```python
from build123d import *

# Parameters (mm, degrees)
BOSS_EXTRUDE1_DEPTH                             = 187.5
CUT_EXTRUDE1_DEPTH                              = 255
CUT_EXTRUDE2_DEPTH                              = 10
SKETCH4_R                                       = 1.5
CUT_EXTRUDE3_DEPTH                              = 255
SKETCH5_R                                       = 1.5
CUT_EXTRUDE4_DEPTH                              = 10
CSK_FOR_M3_FLAT_HEAD_MACHINE_SCREW1_D           = 3.4
CSK_FOR_M3_FLAT_HEAD_MACHINE_SCREW1_CSINK_D     = 6.3
CSK_FOR_M3_FLAT_HEAD_MACHINE_SCREW1_CSINK_ANGLE = 90
CSK_FOR_M3_FLAT_HEAD_MACHINE_SCREW2_D           = 3.4
CSK_FOR_M3_FLAT_HEAD_MACHINE_SCREW2_DEPTH       = 10
CSK_FOR_M3_FLAT_HEAD_MACHINE_SCREW2_CSINK_D     = 6.3
CSK_FOR_M3_FLAT_HEAD_MACHINE_SCREW2_CSINK_ANGLE = 90
CSK_FOR_M3_FLAT_HEAD_MACHINE_SCREW2_TIP         = 1.021463052
CSK_FOR_M3_FLAT_HEAD_MACHINE_SCREW3_D           = 3.4
CSK_FOR_M3_FLAT_HEAD_MACHINE_SCREW3_DEPTH       = 10
CSK_FOR_M3_FLAT_HEAD_MACHINE_SCREW3_CSINK_D     = 6.3
CSK_FOR_M3_FLAT_HEAD_MACHINE_SCREW3_CSINK_ANGLE = 90
CSK_FOR_M3_FLAT_HEAD_MACHINE_SCREW3_TIP         = 1.021463052


with BuildPart() as part:
    # Sketch1 → Boss-Extrude1 (new body, symmetric)
    with BuildSketch(Plane(origin=(0, 0, 0), x_dir=(0, 0, -1), z_dir=(1, 0, 0))):
        with BuildLine():
            Line((125, -45), (127, -45))
            Line((127, -45), (127, -2.5))
            ThreePointArc((127, -2.5), (126.267766953, -0.732233047), (124.5, 0))
            Line((124.5, 0), (-124.5, 0))
            ThreePointArc((-124.5, 0), (-126.267766953, -0.732233047), (-127, -2.5))
            Line((-127, -2.5), (-127, -45))
            Line((-127, -45), (-125, -45))
            Line((-125, -45), (-125, -2.5))
            ThreePointArc((-125, -2.5), (-124.853553391, -2.146446609), (-124.5, -2))
            Line((-124.5, -2), (124.5, -2))
            ThreePointArc((124.5, -2), (124.853553391, -2.146446609), (125, -2.5))
            Line((125, -2.5), (125, -45))
        make_face()
    extrude(amount=BOSS_EXTRUDE1_DEPTH, both=True)

    # Sketch2 → Cut-Extrude1 (cut, through all)
    with BuildSketch(Plane.XY.offset(127)):
        with BuildLine():
            Line((-169.5, -45), (169.5, -45))
            Line((169.5, -45), (169.5, -30))
            ThreePointArc((169.5, -30), (166.571067812, -22.928932188), (159.5, -20))
            Line((159.5, -20), (-159.5, -20))
            ThreePointArc((-159.5, -20), (-166.571067812, -22.928932188), (-169.5, -30))
            Line((-169.5, -30), (-169.5, -45))
        make_face()
    extrude(amount=-CUT_EXTRUDE1_DEPTH, mode=Mode.SUBTRACT)

    # Sketch3 → Cut-Extrude2 (cut)
    with BuildSketch(Plane(origin=(0, 0, 0), x_dir=(1, 0, 0), z_dir=(0, 1, 0))):
        with BuildLine():
            Line((-139.5, 97), (73.5, 97))
            ThreePointArc((73.5, 97), (80.571067812, 94.071067812), (83.5, 87))
            Line((83.5, 87), (83.5, -87))
            ThreePointArc((83.5, -87), (80.571067812, -94.071067812), (73.5, -97))
            Line((73.5, -97), (-139.5, -97))
            ThreePointArc((-139.5, -97), (-146.571067812, -94.071067812), (-149.5, -87))
            Line((-149.5, -87), (-149.5, 87))
            ThreePointArc((-149.5, 87), (-146.571067812, 94.071067812), (-139.5, 97))
        make_face()
    extrude(amount=-CUT_EXTRUDE2_DEPTH, mode=Mode.SUBTRACT)

    # Sketch4 → Cut-Extrude3 (cut, through all)
    with BuildSketch(Plane.XY.offset(127)):
        with Locations((-178.5, -33)):
            Circle(SKETCH4_R)
        with Locations((-166.5, -9)):
            Circle(SKETCH4_R)
        with Locations((166.5, -9)):
            Circle(SKETCH4_R)
        with Locations((178.5, -33)):
            Circle(SKETCH4_R)
    extrude(amount=-CUT_EXTRUDE3_DEPTH, mode=Mode.SUBTRACT)

    # Sketch5 → Cut-Extrude4 (cut)
    with BuildSketch(Plane(origin=(0, 0, 0), x_dir=(1, 0, 0), z_dir=(0, 1, 0))):
        with Locations(Location((-178.5, 118, 0), (0, 0, 270))):  # turned: the seam where the file's is
            Circle(SKETCH5_R)
        with Locations(Location((-154.5, 118, 0), (0, 0, 270))):  # turned: the seam where the file's is
            Circle(SKETCH5_R)
        with Locations(Location((154.5, 118, 0), (0, 0, 270))):  # turned: the seam where the file's is
            Circle(SKETCH5_R)
        with Locations(Location((178.5, 118, 0), (0, 0, 270))):  # turned: the seam where the file's is
            Circle(SKETCH5_R)
        with Locations(Location((178.5, -118, 0), (0, 0, 270))):  # turned: the seam where the file's is
            Circle(SKETCH5_R)
        with Locations(Location((154.5, -118, 0), (0, 0, 270))):  # turned: the seam where the file's is
            Circle(SKETCH5_R)
        with Locations(Location((-178.5, -118, 0), (0, 0, 270))):  # turned: the seam where the file's is
            Circle(SKETCH5_R)
        with Locations(Location((-154.5, -118, 0), (0, 0, 270))):  # turned: the seam where the file's is
            Circle(SKETCH5_R)
        with Locations(Location((88.5, 41.85, 0), (0, 0, 270))):  # turned: the seam where the file's is
            Circle(SKETCH5_R)
        with Locations(Location((88.5, -30.15, 0), (0, 0, 270))):  # turned: the seam where the file's is
            Circle(SKETCH5_R)
        with Locations(Location((125.5, 41.85, 0), (0, 0, 270))):  # turned: the seam where the file's is
            Circle(SKETCH5_R)
        with Locations(Location((125.5, -30.15, 0), (0, 0, 270))):  # turned: the seam where the file's is
            Circle(SKETCH5_R)
        with Locations(Location((-154.5, 28.85, 0), (0, 0, 270))):  # turned: the seam where the file's is
            Circle(SKETCH5_R)
        with Locations(Location((-173.5, 28.85, 0), (0, 0, 270))):  # turned: the seam where the file's is
            Circle(SKETCH5_R)
        with Locations(Location((-173.5, 4.85, 0), (0, 0, 270))):  # turned: the seam where the file's is
            Circle(SKETCH5_R)
        with Locations(Location((-154.5, 4.85, 0), (0, 0, 270))):  # turned: the seam where the file's is
            Circle(SKETCH5_R)
        with Locations(Location((-154.5, -42.15, 0), (0, 0, 270))):  # turned: the seam where the file's is
            Circle(SKETCH5_R)
        with Locations(Location((-173.5, -42.15, 0), (0, 0, 270))):  # turned: the seam where the file's is
            Circle(SKETCH5_R)
        with Locations(Location((-166.5, 82.25, 0), (0, 0, 270))):  # turned: the seam where the file's is
            Circle(SKETCH5_R)
        with Locations(Location((-154.5, 82.25, 0), (0, 0, 270))):  # turned: the seam where the file's is
            Circle(SKETCH5_R)
        with Locations(Location((-166.5, 44.25, 0), (0, 0, 270))):  # turned: the seam where the file's is
            Circle(SKETCH5_R)
        with Locations(Location((-154.5, 44.25, 0), (0, 0, 270))):  # turned: the seam where the file's is
            Circle(SKETCH5_R)
    extrude(amount=-CUT_EXTRUDE4_DEPTH, mode=Mode.SUBTRACT)

    # CSK for M3 Flat Head Machine Screw1 (through all)
    with Locations(Plane(origin=(0, 0, 0), x_dir=(-1, 0, 0), z_dir=(0, 1, 0))):
        with Locations((154.5, 118), (178.5, 118), (154.5, 42.15), (173.5, 42.15), (154.5, -4.85), (173.5, -4.85), (173.5, -28.85), (154.5, -28.85), (154.5, -44.25), (166.5, -44.25), (166.5, -82.25), (154.5, -82.25), (178.5, -118), (154.5, -118), (-154.5, -118), (-178.5, -118), (-125.5, -41.85), (-88.5, -41.85), (-125.5, 30.15), (-88.5, 30.15), (-178.5, 118), (-154.5, 118)):
            CounterSinkHole(CSK_FOR_M3_FLAT_HEAD_MACHINE_SCREW1_D / 2, CSK_FOR_M3_FLAT_HEAD_MACHINE_SCREW1_CSINK_D / 2, counter_sink_angle=CSK_FOR_M3_FLAT_HEAD_MACHINE_SCREW1_CSINK_ANGLE)

    # CSK for M3 Flat Head Machine Screw2
    with Locations(Plane.XY.offset(127)):
        with Locations((166.5, -9), (178.5, -33), (-178.5, -33), (-166.5, -9)):
            CounterSinkHole(CSK_FOR_M3_FLAT_HEAD_MACHINE_SCREW2_D / 2, CSK_FOR_M3_FLAT_HEAD_MACHINE_SCREW2_CSINK_D / 2, depth=CSK_FOR_M3_FLAT_HEAD_MACHINE_SCREW2_DEPTH, counter_sink_angle=CSK_FOR_M3_FLAT_HEAD_MACHINE_SCREW2_CSINK_ANGLE)
            with Locations((0, 0, -(CSK_FOR_M3_FLAT_HEAD_MACHINE_SCREW2_DEPTH + CSK_FOR_M3_FLAT_HEAD_MACHINE_SCREW2_TIP / 2))):  # 118° drill point
                Cone(0, CSK_FOR_M3_FLAT_HEAD_MACHINE_SCREW2_D / 2, CSK_FOR_M3_FLAT_HEAD_MACHINE_SCREW2_TIP, mode=Mode.SUBTRACT)

    # CSK for M3 Flat Head Machine Screw3
    with Locations(Plane(origin=(0, 0, -127), x_dir=(-1, 0, 0), z_dir=(0, 0, -1))):
        with Locations((-166.5, -9), (178.5, -33), (166.5, -9), (-178.5, -33)):
            CounterSinkHole(CSK_FOR_M3_FLAT_HEAD_MACHINE_SCREW3_D / 2, CSK_FOR_M3_FLAT_HEAD_MACHINE_SCREW3_CSINK_D / 2, depth=CSK_FOR_M3_FLAT_HEAD_MACHINE_SCREW3_DEPTH, counter_sink_angle=CSK_FOR_M3_FLAT_HEAD_MACHINE_SCREW3_CSINK_ANGLE)
            with Locations((0, 0, -(CSK_FOR_M3_FLAT_HEAD_MACHINE_SCREW3_DEPTH + CSK_FOR_M3_FLAT_HEAD_MACHINE_SCREW3_TIP / 2))):  # 118° drill point
                Cone(0, CSK_FOR_M3_FLAT_HEAD_MACHINE_SCREW3_D / 2, CSK_FOR_M3_FLAT_HEAD_MACHINE_SCREW3_TIP, mode=Mode.SUBTRACT)


solid = part.part
```
Verification items for the finished model (mm, model axes). A direction names the side the tool comes from. Coordinates: 2 decimals unless noted, no trailing zeros. Loops run counter-clockwise (first coordinate to the right, second up) from the corner with the lowest first, then second, coordinate; pieces in that order, holes last. Notation, with made-up numbers: (75.5, 7.25) - (85.5, 7.25) arc R21 ccw to (85.5, 17.25) - close; hole circle Ø7 at (36.25, 28.5). An arc over 180 degrees is marked (long way). Answer as a JSON object with one key per item and string values.
(1) Access from +Z, -Z, +X, -X, +Y, -Y to the whole of each face (thin tool, end or side, straight path). Record for faces 4 (the flat face through (3, -14, -125)), 5 (the cylindrical face through (80.65, -0.99, 93.99)), 6 (the cylindrical face through (-166.49, -22.85, -125.99)), 7 (the flat face through (3, -14, 127)), 8 (the flat face through (86, 0, -2)).
Response:
{"face 4": "+X, -X, -Y", "face 5": "+Y, -Y", "face 6": "+Z, -Z, -Y", "face 7": "+Z, +X, -X, +Y, -Y", "face 8": "+Z, -Z, +X, -X, +Y"}
(2) Cross-section at C-C, the plane y = -26. Record the boundary of the cut face in (x, z), then the cut area to 3 significant figures.
Response:
{"outline": "(-187.5, -127) - (-168.67, -127) - (-168.67, -125) - (-187.5, -125) - close; (-187.5, 125) - (-168.67, 125) - (-168.67, 127) - (-187.5, 127) - close; (168.67, -127) - (187.5, -127) - (187.5, -125) - (168.67, -125) - close; (168.67, 125) - (187.5, 125) - (187.5, 127) - (168.67, 127) - close", "area": "151 mm²"}
(3) Mould release check, pull along X, two halves, no side actions. Record for faces 1 (the flat face through (187.5, -1, 1)), 2 (the cylindrical face through (-166.49, -22.85, 126.01)), 3 (the flat face through (-187.5, -1, 1)): pulls with the +X half, pulls with the -X half, needs draft (parallel to the pull), parting line crosses it, or undercut.
Response:
{"face 1": "pulls with the +X half", "face 2": "undercut", "face 3": "pulls with the -X half"}
(4) Cross-section at B-B, the plane x = 41. Record the boundary of the cut face in (y, z).
Response:
{"outline": "(-20, -127) - (-2.5, -127) arc R2.5 ccw to (0, -124.5) - (0, -97) - (-2, -97) - (-2, -124.5) arc R0.5 cw to (-2.5, -125) - (-20, -125) - close; (-20, 125) - (-2.5, 125) arc R0.5 cw to (-2, 124.5) - (-2, 97) - (0, 97) - (0, 124.5) arc R2.5 ccw to (-2.5, 127) - (-20, 127) - close"}
(5) Cross-section at A-A, the plane z = 7. Record the boundary of the cut face in (x, y), then the cut area to 3 significant figures.
Response:
{"outline": "(-187.5, -2) - (-149.5, -2) - (-149.5, 0) - (-187.5, 0) - close; (83.5, -2) - (187.5, -2) - (187.5, 0) - (83.5, 0) - close", "area": "284 mm²"}
(6) Cross-section at D-D, the plane x = 113. Record the boundary of the cut face in (y, z), then the cut area to 3 significant figures.
Response:
{"outline": "(-20, -127) - (-2.5, -127) arc R2.5 ccw to (0, -124.5) - (0, 124.5) arc R2.5 ccw to (-2.5, 127) - (-20, 127) - (-20, 125) - (-2.5, 125) arc R0.5 cw to (-2, 124.5) - (-2, -124.5) arc R0.5 cw to (-2.5, -125) - (-20, -125) - close", "area": "577 mm²"}
(7) Scan lines: line 1 along X through (y, z) = (-1.7, 42.15); line 2 along X through (y, z) = (-1.9, -82.25); line 3 along X through (y, z) = (-1.55, -118). Record each from-to range of solid material in increasing order.
Response:
{"line 1": "x = -187.5 to -175.2, -171.8 to -156.2, -152.8 to -149.5, 83.5 to 187.5", "line 2": "x = -187.5 to -168.2, -164.8 to -156.2, -152.8 to -149.5, 83.5 to 187.5", "line 3": "x = -187.5 to -180.2, -176.8 to -156.2, -152.8 to 152.8, 156.2 to 176.8, 180.2 to 187.5"}
(8) Go/stop test with flat-tipped pins: pin 1 Ø5.5 at (x, z) = (178.5, 118) entering from -Y; pin 2 Ø5.5 at (x, z) = (-154.5, -82.25) entering from +Y; pin 3 Ø1 at (x, y) = (-76.5, -0.5) entering from -Z. Record where each tip stops, or that it passes through.
Response:
{"pin 1": "stops at y = -2", "pin 2": "stops at y = -0.4", "pin 3": "stops at z = -126.5"}
